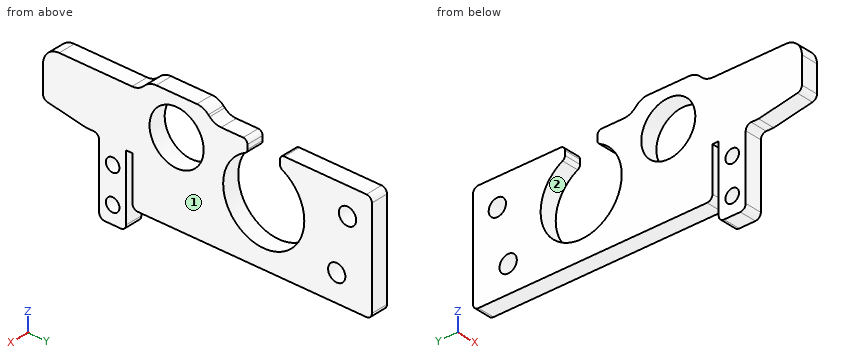
from build123d import *

# Parameters (mm, degrees)
SKETCH1_R           = 5
SKETCH1_R_2         = 1.6
SKETCH1_R_3         = 1.25
BOSS_EXTRUDE1_DEPTH = 3.18
CHAMFER1_SIZE       = 8
CHAMFER1_SIZE2      = 1.410615846
FILLET1_R           = 1
FILLET2_R           = 3
CUT_EXTRUDE5_DEPTH  = 66.452032054
FILLET3_R           = 0.8


with BuildPart() as part:
    # Sketch1 → Boss-Extrude1 (new body)
    with BuildSketch(Plane(origin=(0, 0, 0), x_dir=(0, 0, -1), z_dir=(1, 0, 0))):
        Polygon((0, 0), (0, 17.7), (-2, 19.7), (-2, 29.7), (0, 31.7), (0, 60.81), (20, 60.81), (20, 16.53), (10.85, 16.53), (10.85, 15.38), (24, 15.38), (24, 10.38), (10.17, 10.38), (10.17, 0), align=None)
        with Locations(Location((5, 24.7, 0), (0, 0, 180))):
            Circle(SKETCH1_R, mode=Mode.SUBTRACT)
        with Locations(Location((5, 56.31, 0), (0, 0, 180))):
            Circle(SKETCH1_R_2, mode=Mode.SUBTRACT)
        with Locations(Location((15, 54.31, 0), (0, 0, 180))):
            Circle(SKETCH1_R_2, mode=Mode.SUBTRACT)
        with Locations(Location((20.75, 12.88, 0), (0, 0, 180))):
            Circle(SKETCH1_R_3, mode=Mode.SUBTRACT)
        with Locations(Location((14.25, 12.88, 0), (0, 0, 180))):
            Circle(SKETCH1_R_3, mode=Mode.SUBTRACT)
    extrude(amount=BOSS_EXTRUDE1_DEPTH)

    # Chamfer1
    chamfer1_edges = [part.edges().sort_by_distance(p)[0] for p in [
        (1.59, 0, -10.17),
    ]]
    chamfer1_side = [part.faces().sort_by_distance(p)[0] for p in [
        (1.59, 5.19, -10.17),
    ]]
    chamfer(chamfer1_edges, length=CHAMFER1_SIZE, length2=CHAMFER1_SIZE2, reference=chamfer1_side[0])

    # Fillet1
    fillet1_edges = [part.edges().sort_by_distance(p)[0] for p in [
        (1.59, 60.81, 0),
        (1.59, 60.81, -20),
        (1.59, 16.53, -20),
        (1.59, 15.38, -24),
        (1.59, 10.38, -24),
        (1.59, 10.38, -10.17),
        (1.59, 0, -8.759384154),
    ]]
    fillet(fillet1_edges, radius=FILLET1_R)

    # Fillet2
    fillet2_edges = [part.edges().sort_by_distance(p)[0] for p in [
        (1.59, 0, 0),
        (1.59, 17.7, 0),
        (1.59, 19.7, 2),
        (1.59, 29.7, 2),
        (1.59, 31.7, 0),
    ]]
    fillet(fillet2_edges, radius=FILLET2_R)

    # Sketch8 → Cut-Extrude5 (cut, through all)
    with BuildSketch(Plane(origin=(3.18, 0, 0), x_dir=(0, 0, -1), z_dir=(1, 0, 0))):
        with BuildLine():
            Line((0, 43.810865899), (2.126136458, 43.810865899))
            ThreePointArc((2.126136458, 43.810865899), (16.5, 40.810865899), (2.126136458, 37.810865899))
            Line((2.126136458, 37.810865899), (0, 37.810865899))
            Line((0, 37.810865899), (0, 43.810865899))
        make_face()
    extrude(amount=-CUT_EXTRUDE5_DEPTH, mode=Mode.SUBTRACT)

    # Fillet3
    fillet3_edges = [part.edges().sort_by_distance(p)[0] for p in [
        (1.59, 37.810865899, 0),
        (1.59, 43.810865899, 0),
        (1.59, 43.810865899, -2.126136458),
        (1.59, 37.810865899, -2.126136458),
    ]]
    fillet(fillet3_edges, radius=FILLET3_R)


solid = part.part
Geometry: final body of the model. Coordinates: model frame, mm. Face numbers are marked on the shaded views. Round coordinates to 2 decimals unless told otherwise and drop trailing zeros. Loops run counter-clockwise (first coordinate to the right, second up) from the corner with the lowest first, then second, coordinate; pieces in that order, holes last.
Q1. Material intervals for L1, parallel to Z at x = 1.55, y = 54.31; L2, parallel to Y at x = 1.2, z = -15; L3, parallel to Y at x = 1.6, z = -5, sorted ascending.
Q2. Section C-C on z = -4. Return loops of the section in (x, y).
Q3. Pull-direction query (Z, two-part tool) for the marked faces 1 and 2; classes: released by +Z, released by -Z, zero draft, split by the parting line, or undercut.
Q4. Section A-A on z = -20.75. Return loops of the section in (x, y), plus the area to 3 significant figures.
Q5. Section B-B on y = 47. Return loops of the section in (x, z), plus the area to 3 significant figures.
Q6. Pin query (flat end, axial travel): P1, Ø1.3, axis at x = 1.5, y = 15.5, coming from the -Z side; P2, Ø1, axis at x = 1.5, y = 28.5, coming from the -Z side; P3, Ø1.1, axis at x = 1, y = 9, coming from the -Z side; P4, Ø12, axis at y = 40.81, z = -9, coming from the -X side. Return the tip coordinate at first contact, or that it passes through.
Q7. Section D-D on x = 0.65. State how many separate pieces and enclosed holes the cut face has, plus the area to 3 significant figures.
Evaluation:
1. L1: z = -20 to -16.6, -13.4 to 0
1. L2: y = 10.38 to 11.88, 13.88 to 15.38, 16.53 to 36.31, 45.31 to 52.71, 55.91 to 60.81
1. L3: y = 0 to 19.7, 29.7 to 34.47, 47.16 to 54.71, 57.91 to 60.81
2. outline: (0, 0) - (3.18, 0) - (3.18, 19.8) - (0, 19.8) - close; (0, 29.6) - (3.18, 29.6) - (3.18, 35.22) - (0, 35.22) - close; (0, 46.4) - (3.18, 46.4) - (3.18, 55.06) - (0, 55.06) - close; (0, 57.56) - (3.18, 57.56) - (3.18, 60.81) - (0, 60.81) - close
3. face 1: zero draft
3. face 2: undercut
4. outline: (0, 10.38) - (3.18, 10.38) - (3.18, 11.63) - (0, 11.63) - close; (0, 14.13) - (3.18, 14.13) - (3.18, 15.38) - (0, 15.38) - close
4. area: 7.95 mm2
5. outline: (0, -20) - (3.18, -20) - (3.18, -13.24) - (0, -13.24) - close; (0, -4.76) - (3.18, -4.76) - (3.18, 0) - (0, 0) - close
5. area: 36.7 mm2
6. P1: stops at z = -23.88
6. P2: stops at z = -20
6. P3: stops at z = -10.18
6. P4: passes through
7. separate pieces: 1
7. enclosed holes: 5
7. area: 847 mm2
